Can you work these out from the model? Positions are in its coordinate system, mm. Round coordinates to 2 decimals unless told otherwise and drop trailing zeros. Write each loop counter-clockwise with the first axis right and the second up, starting at its lowest first coordinate (ties: lowest second). Pieces come first, ordered by that corner, then holes.
Q1. If we section it at B-B (x = 0): Please give me the cut outline in (y, z), plus the area to 3 significant figures.
Q2. If we section it at D-D (x = 25): Please give me the cut outline in (y, z).
Q3. I'm going to push flat-ended pins straight in: pin 1 Ø1 at (y, z) = (-1, 1) entering from -X; pin 2 Ø24 at (x, y) = (0, 0) entering from -Z; pin 3 Ø10 at (x, y) = (0, 25) entering from +Z; pin 4 Ø1 at (x, z) = (27, 1.5) entering from -Y. Where does each tip first touch, or does it pass through?
Q4. Please list where these lines run through material, in increasing order: line 1 along Y through (x, z) = (0, 0.8); line 2 along X through (y, z) = (-3.5, 1.1); line 3 along X through (y, z) = (-26, 0.65).
Q5. If we section it at C-C (y = -25): Please give me the cut outline in (x, z).
Q6. If we section it at A-A (z = 0.5): Please give me the cut outline in (x, y).
from build123d import *

# Parameters (mm, degrees)
MODEL_R             = 5.5
MODEL_R_2           = 7.5
BOSS_EXTRUDE1_DEPTH = 2


with BuildPart() as part:
    # Model → Boss-Extrude1 (new body)
    with BuildSketch(Plane.XY):
        with BuildLine():
            Line((8.947329511, -33.697448784), (10.207027791, -37.122319212))
            ThreePointArc((10.207027791, -37.122319212), (-7.201532375, -37.820469741), (-23.135313057, -30.773483549))
            Line((-23.135313057, -30.773483549), (-20.68154198, -27.990692072))
            ThreePointArc((-20.68154198, -27.990692072), (-20.947588277, -23.756401179), (-25.18187917, -24.022447477))
            Line((-25.18187917, -24.022447477), (-27.635650248, -26.805238954))
            ThreePointArc((-27.635650248, -26.805238954), (-38.49998136, -0.037885337), (-27.688351274, 26.750798188))
            Line((-27.688351274, 26.750798188), (-25.246259349, 23.992215172))
            ThreePointArc((-25.246259349, 23.992215172), (-21.011453059, 23.734502765), (-20.753740651, 27.969309055))
            Line((-20.753740651, 27.969309055), (-23.195832576, 30.727892071))
            ThreePointArc((-23.195832576, 30.727892071), (-7.250949904, 37.811026507), (10.183062279, 37.128900369))
            Line((10.183062279, 37.128900369), (8.940382065, 33.678361242))
            ThreePointArc((8.940382065, 33.678361242), (10.746378971, 29.839375176), (14.585365036, 31.645372081))
            Line((14.585365036, 31.645372081), (15.82804525, 35.095911209))
            ThreePointArc((15.82804525, 35.095911209), (38.499997976, 0.012482786), (15.85080009, -35.085640033))
            Line((15.85080009, -35.085640033), (14.578417591, -31.626283722))
            ThreePointArc((14.578417591, -31.626283722), (10.72729102, -29.846322213), (8.947329511, -33.697448784))
        make_face()
        with Locations((-25, 0)):
            Circle(MODEL_R, mode=Mode.SUBTRACT)
        with Locations((0, 25)):
            Circle(MODEL_R, mode=Mode.SUBTRACT)
        with Locations((0, -25)):
            Circle(MODEL_R, mode=Mode.SUBTRACT)
        with Locations((25, 0)):
            Circle(MODEL_R, mode=Mode.SUBTRACT)
        Circle(MODEL_R_2, mode=Mode.SUBTRACT)
    extrude(amount=BOSS_EXTRUDE1_DEPTH)


solid = part.part
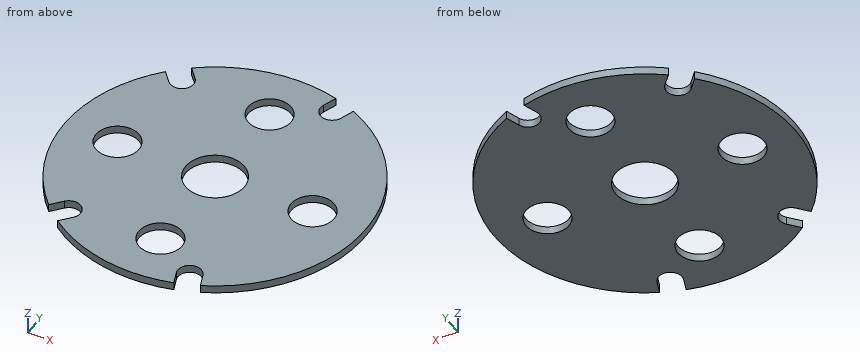
A:
1. outline: (-38.5, 0) - (-30.5, 0) - (-30.5, 2) - (-38.5, 2) - close; (-19.5, 0) - (-7.5, 0) - (-7.5, 2) - (-19.5, 2) - close; (7.5, 0) - (19.5, 0) - (19.5, 2) - (7.5, 2) - close; (30.5, 0) - (38.5, 0) - (38.5, 2) - (30.5, 2) - close
1. area: 80.0 mm2
2. outline: (-29.28, 0) - (-5.5, 0) - (-5.5, 2) - (-29.28, 2) - close; (5.5, 0) - (29.28, 0) - (29.28, 2) - (5.5, 2) - close
3. pin 1: stops at x = -38.5
3. pin 2: stops at z = 0
3. pin 3: passes through
3. pin 4: stops at y = -27.93
4. line 1: y = -38.5 to -30.5, -19.5 to -7.5, 7.5 to 19.5, 30.5 to 38.5
4. line 2: x = -38.34 to -29.24, -20.76 to -6.63, 6.63 to 20.76, 29.24 to 38.34
4. line 3: x = -28.39 to -26.93, -19.93 to -5.41, 5.41 to 28.39
5. outline: (-29.28, 0) - (-26.04, 0) - (-26.04, 2) - (-29.28, 2) - close; (-20.11, 0) - (-5.5, 0) - (-5.5, 2) - (-20.11, 2) - close; (5.5, 0) - (29.28, 0) - (29.28, 2) - (5.5, 2) - close
6. outline: (-27.69, 26.75) arc R38.5 ccw to (-27.64, -26.81) - (-25.18, -24.02) arc R3 cw to (-20.68, -27.99) - (-23.14, -30.77) arc R38.5 ccw to (10.21, -37.12) - (8.95, -33.7) arc R3 cw to (14.58, -31.63) - (15.85, -35.09) arc R38.5 ccw to (15.83, 35.1) - (14.59, 31.65) arc R3 cw to (8.94, 33.68) - (10.18, 37.13) arc R38.5 ccw to (-23.2, 30.73) - (-20.75, 27.97) arc R3 cw to (-25.25, 23.99) - close; hole circle Ø11 at (-25, 0); hole circle Ø15 at (0, 0); hole circle Ø11 at (0, -25); hole circle Ø11 at (0, 25); hole circle Ø11 at (25, 0)
